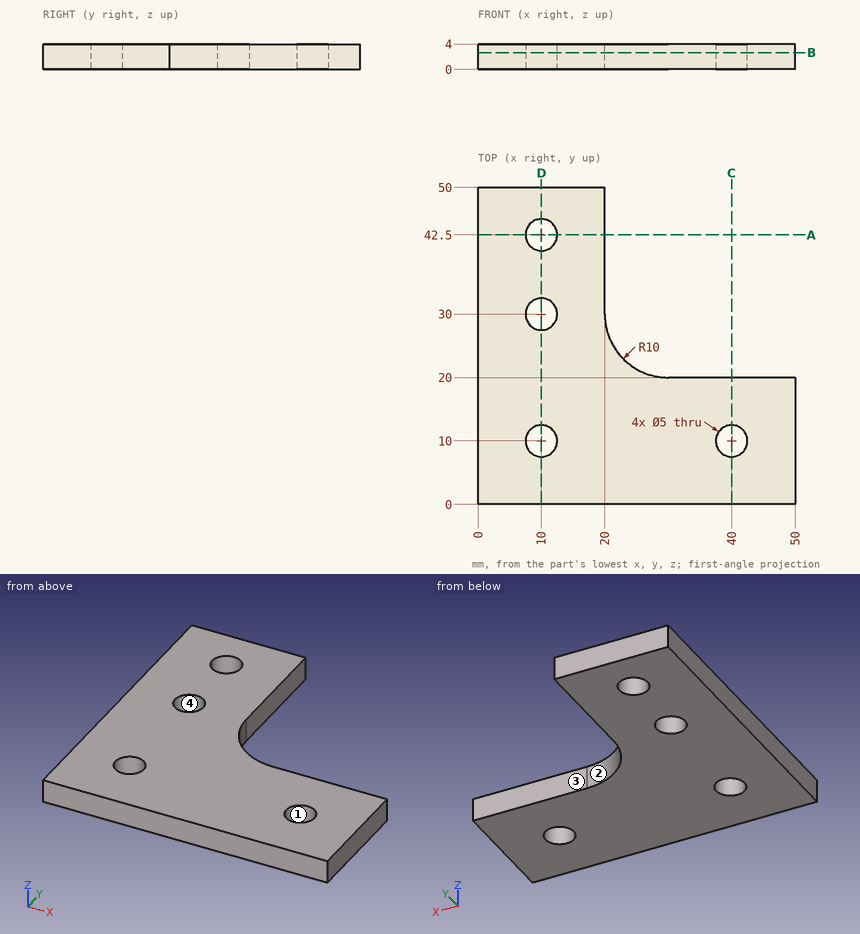
Geometry check sheet. Reference: drawing and pictorial views, mm from the part's lowest x, y, z. Round coordinates to 2 decimals unless told otherwise and drop trailing zeros. Write each loop counter-clockwise with the first axis right and the second up, starting at its lowest first coordinate (ties: lowest second). Pieces come first, ordered by that corner, then holes. Notation, with made-up numbers: (70, -15.5) -> (94, -15.5) arc R15 cw to (94, -10.5) -> close; hole circle Ø4 at (-2.5, 83.25). An arc over 180 degrees is marked (long way). One line per question, with ' | ' between items. Start each with the question number.
1. Release check for a two-part mould opening along X. For the marked faces 1, 2, 3 and 4 record: +X half, -X half, draft (parallel to the pull), parting line (faces both ways), or undercut.
2. Sectioned sample at A-A, the plane y = 42.5. Record the cut outline in (x, z).
3. Sectioned sample at B-B, the plane z = 2.65. Record the cut outline in (x, y), then the cut area to 3 significant figures.
4. Sectioned sample at D-D, the plane x = 10. Record the cut outline in (y, z), then the cut area to 3 significant figures.
5. Scan lines: line 1 along Y through (x, z) = (10, 0.95); line 2 along Y through (x, z) = (40, 0.9); line 3 along X through (y, z) = (12, 1.6). Record each from-to range of solid material in increasing order. Write a range as from..to.
6. Depth check by flat-ended pin: pin 1 (2 mm diameter, centred on x = 38, z = 1.5, fed in from +Y); pin 2 (3 mm diameter, centred on x = 10, y = 30, fed in from +Z). Enter the tip coordinate at first touch or a pass-through.
Taken from the geometry:
1) face 1: undercut | face 2: +X half | face 3: draft | face 4: undercut
2) outline: (0, 0) -> (7.5, 0) -> (7.5, 4) -> (0, 4) -> close; (12.5, 0) -> (20, 0) -> (20, 4) -> (12.5, 4) -> close
3) outline: (0, 0) -> (50, 0) -> (50, 20) -> (30, 20) arc R10 cw to (20, 30) -> (20, 50) -> (0, 50) -> close; hole circle Ø5 at (10, 10); hole circle Ø5 at (10, 30); hole circle Ø5 at (10, 42.5); hole circle Ø5 at (40, 10) | area: 1,540 mm^2
4) outline: (0, 0) -> (7.5, 0) -> (7.5, 4) -> (0, 4) -> close; (12.5, 0) -> (27.5, 0) -> (27.5, 4) -> (12.5, 4) -> close; (32.5, 0) -> (40, 0) -> (40, 4) -> (32.5, 4) -> close; (45, 0) -> (50, 0) -> (50, 4) -> (45, 4) -> close | area: 140 mm^2
5) line 1: y = 0..7.5, 12.5..27.5, 32.5..40, 45..50 | line 2: y = 0..7.5, 12.5..20 | line 3: x = 0..8.5, 11.5..38.5, 41.5..50
6) pin 1: stops at y = 20 | pin 2: passes through
